Source: CAD feature listing. Evaluate the final solid. Frame: model axes, mm. A direction names the side the tool comes from. Give positions to 0.01 mm unless a question says otherwise; leave off trailing zeros. Order: outer loops, then holes, each group sorted by start corner. A loop starts at its lowest first (then second) coordinate and runs counter-clockwise, first axis right, second up.
1) Section A-A, the plane y = -23.5. Return loops of the section in (x, z).
2) Draft query along X for faces 4 (the face through (-14.5, -1, 5)), 5 (the face through (20, -1, 4)), 6 (the face through (-13, 1, 8)). Return one class per face: released by +X, released by -X, zero draft, split by the parting line, or undercut.
3) Access query for faces 1 (the face through (0, -5.795, 14)), 2 (the face through (0, 1, 0)), 3 (the face through (6.622, 0, 14)). Directions: +Z, -Z, +X, -X, +Y, -Y. A direction counts if a zero-diameter tool reaches every point of the face in a straight line with its end or side. Return the directions, or none.
4) Section D-D, the plane x = 10. Return loops of the section in (y, z).
5) Section C-C, the plane z = 10.5. Return loops of the section in (x, y), plus the area to 3 significant figures.
6) First-contact query: P1, Ø3.5, axis at x = -15.5, y = 14.5, coming from the +Z side; P2, Ø12.5, axis at y = -2, z = 22.5, coming from the -X side; P3, Ø1, axis at x = 7, z = 29.5, coming from the +Y side. Flat tips, straight axial feed; report the tip coordinate or a pass-through.
7) Material intervals for line 1 (X direction, y = -32, z = 5.5); line 2 (Y direction, x = -5, z = 10.5); line 3 (Z direction, x = -16, y = -47.5), sorted ascending.
8) Section B-B, the plane x = -4. Return loops of the section in (y, z).
```python
from build123d import *

# Parameters (mm, degrees)
F0_W     = 40
F0_H     = 111
F1_DEPTH = 3
F2_W     = 2.5
F2_H     = 111
F3_DEPTH = 5
F5_W     = 13.24492
F5_H     = 11.589288
F6_DEPTH = 30
F8_DEPTH = 25.4


with BuildPart() as f1:
    # F0 (on Top) → F1 (new body)
    with BuildSketch(Plane.XY):
        Rectangle(F0_W, F0_H)
    extrude(amount=F1_DEPTH)

    # F2 (on face) → F3 (join)
    with BuildSketch(Plane.XY.offset(3)):
        with Locations((-13.25, 0)):
            Rectangle(F2_W, F2_H)
        with Locations((-18.75, 0)):
            Rectangle(F2_W, F2_H)
    extrude(amount=F3_DEPTH)

    # F4: F1 across plane


with BuildPart() as f1_1:
    add(f1.part)
    add(f1.part.mirror(Plane.YZ))

    # F5 (on face) → F6 (join)
    with BuildSketch(Plane.XY.offset(3)):
        Rectangle(F5_W, F5_H)
    extrude(amount=F6_DEPTH)

    # F7 (on face) → F8 (cut)
    with BuildSketch(Plane(origin=(-6.62246, 0, 0), x_dir=(0, -1, 0), z_dir=(-1, 0, 0))):
        Polygon((5.794644, 33), (-5.794644, 33), (5.794644, 24.885093), align=None)
    extrude(amount=-F8_DEPTH, mode=Mode.SUBTRACT)


solid = f1_1.part
```
From the geometry:
1. outline: (-20, 0) - (20, 0) - (20, 8) - (17.5, 8) - (17.5, 3) - (14.5, 3) - (14.5, 8) - (12, 8) - (12, 3) - (-12, 3) - (-12, 8) - (-14.5, 8) - (-14.5, 3) - (-17.5, 3) - (-17.5, 8) - (-20, 8) - close
2. face 4: undercut
2. face 5: released by +X
2. face 6: zero draft
3. face 1: +Z, -Y
3. face 2: -Z, +X, -X, +Y, -Y
3. face 3: +Z, +Y, -Y
4. outline: (-55.5, 0) - (55.5, 0) - (55.5, 3) - (-55.5, 3) - close
5. outline: (-6.62, -5.79) - (6.62, -5.79) - (6.62, 5.79) - (-6.62, 5.79) - close
5. area: 153 mm2
6. P1: stops at z = 8
6. P2: stops at x = -6.62
6. P3: stops at y = 5.79
7. line 1: x = -20 to -17.5, -14.5 to -12, 12 to 14.5, 17.5 to 20
7. line 2: y = -5.79 to 5.79
7. line 3: z = 0 to 3
8. outline: (-55.5, 0) - (55.5, 0) - (55.5, 3) - (5.79, 3) - (5.79, 33) - (-5.79, 24.89) - (-5.79, 3) - (-55.5, 3) - close
